```python
from build123d import *

# Parameters (mm, degrees)
F0_W     = 152.4
F0_H     = 76.2
F0_R     = 3.5687
F1_DEPTH = 9.525


with BuildPart() as f1:
    # F0 (on Front) → F1 (new body)
    with BuildSketch(Plane.XZ):
        with Locations((-16.148576, -16.968202)):
            Rectangle(F0_W, F0_H)
        with Locations((-79.648576, -42.368202)):
            Circle(F0_R, mode=Mode.SUBTRACT)
        with Locations((47.351424, -42.368202)):
            Circle(F0_R, mode=Mode.SUBTRACT)
        with Locations((-79.648576, 8.431798)):
            Circle(F0_R, mode=Mode.SUBTRACT)
        Polygon((-26.268572, -13.187168), (-15.679849, -6.17511), (-5.738891, -14.078739), (-10.183763, -25.975507), (-22.871804, -25.424486), align=None, mode=Mode.SUBTRACT)
        with Locations((47.351424, 8.431798)):
            Circle(F0_R, mode=Mode.SUBTRACT)
    extrude(amount=F1_DEPTH)


solid = f1.part
```
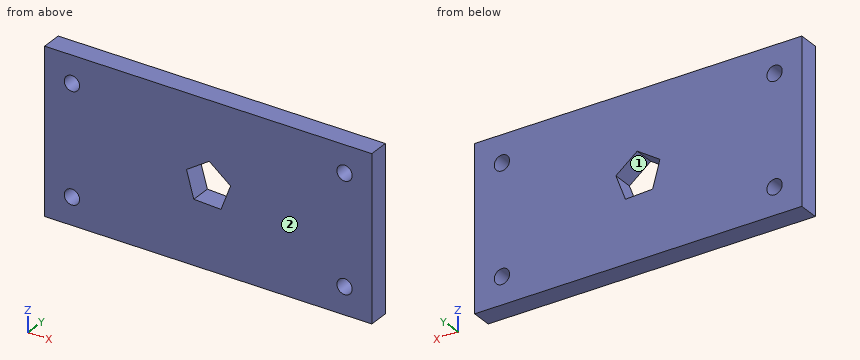
Part model, mm, in its own coordinate system. Face numbers are marked on the shaded views. A direction names the side the tool comes from. Give positions to 0.01 mm unless a question says otherwise; leave off trailing zeros. Order: outer loops, then holes, each group sorted by start corner. A loop starts at its lowest first (then second) coordinate and runs counter-clockwise, first axis right, second up. Notation, with made-up numbers: M -25,-17 L 10,-17 A18 cw 10,-10 Z; hole C 86.25,25.5 d1. An arc over 180 degrees is marked long. Use a Markdown table: item, result. Add a question column.
(1) Probe line 1 along Z through (x, y) = (49.5, -4.75); line 2 along X through (y, z) = (-2, -23); line 3 along Z through (x, y) = (-77, -4.5). List the from-to ranges inside material, lowest first. Write a range as [from, to].
(2) Drop a flat-ended pin along its axis: P1, Ø12, axis at x = -74, z = -20, coming from the +Y side. Give the stop position or say it passes through.
(3) Saw through at B-B, the plane x = 48. Give the cut face in (y, z) (3 decimals), and give its area (3 significant figures).
(4) Saw through at C-C, the plane y = -5.25. Give the cut face in (x, z).
(5) Saw through at A-A, the plane z = -19.5. Give the cut face in (x, y) (3 decimals).
(6) 3-axis set-ups, long thin cutter, end or side, ignore diameter. For the marked faces 1 and 2: which of +Z, -Z, +X, -X, +Y, -Y reach the whole face in a straight line?
(7) Saw through at D-D, the plane z = -41. Give the cut face in (x, y) (3 decimals), and give its area (3 significant figures).
Answer key:
| question | item | result |
|---|---|---|
| 1 | line 1 | [-55.07, -45.22], [-39.52, 5.58], [11.28, 21.13] |
| 1 | line 2 | [-92.35, -23.54], [-9.07, 60.05] |
| 1 | line 3 | [-55.07, -44.76], [-39.98, 6.04], [10.82, 21.13] |
| 2 | P1 | y = 0 |
| 3 | outline | M -9.525,-55.068 L 0,-55.068 L 0,-45.877 L -9.525,-45.877 Z; M -9.525,-38.859 L 0,-38.859 L 0,4.923 L -9.525,4.923 Z; M -9.525,11.941 L 0,11.941 L 0,21.132 L -9.525,21.132 Z |
| 3 | area | 592 mm^2 |
| 4 | outline | M -92.35,-55.07 L 60.05,-55.07 L 60.05,21.13 L -92.35,21.13 Z; hole C -79.65,-42.37 d7.14; hole C -79.65,8.43 d7.14; hole M -26.27,-13.19 L -22.87,-25.42 L -10.18,-25.98 L -5.74,-14.08 L -15.68,-6.18 Z; hole C 47.35,-42.37 d7.14; hole C 47.35,8.43 d7.14 |
| 5 | outline | M -92.349,-9.525 L -24.516,-9.525 L -24.516,0 L -92.349,0 Z; M -7.764,-9.525 L 60.051,-9.525 L 60.051,0 L -7.764,0 Z |
| 6 | face 1 | +Y, -Y |
| 6 | face 2 | +Z, -Z, +X, -X, -Y |
| 7 | outline | M -92.349,-9.525 L -82.945,-9.525 L -82.945,0 L -92.349,0 Z; M -76.353,-9.525 L 44.055,-9.525 L 44.055,0 L -76.353,0 Z; M 50.647,-9.525 L 60.051,-9.525 L 60.051,0 L 50.647,0 Z |
| 7 | area | 1,330 mm^2 |
